For this review, take the finished solid that the model builds, in its own axes (mm). Face numbers are marked on the shaded views. A direction names the side the tool comes from. Give positions to 0.01 mm unless a question says otherwise; leave off trailing zeros. Order: outer loops, then holes, each group sorted by start corner. A loop starts at its lowest first (then second) coordinate and runs counter-clockwise, first axis right, second up. Notation, with made-up numbers: (78, -37.5) -> (96, -37.5) arc R29 ccw to (96, -1.5) -> close; hole circle Ø4 at (36.5, 63.25). An arc over 180 degrees is marked (long way). Return JSON: item names as keys, results as strings. Group by question number.
1) The part is to be moulded in two halves that separate along Y. For the marked faces 6, 7 and 8, say which applies: released by +Y, released by -Y, zero draft, split by the parting line, or undercut.
2) Add section B-B (x = -2.5). Give the boundary of the cut face in (y, z).
3) Add section D-D (y = 15). Give the boundary of the cut face in (x, z), then the cut area to 3 significant figures.
4) For the marked faces 1, 2, 3, 4 and 5, list the 3-axis set-ups (+Z, -Z, +X, -X, +Y, -Y) from which the entire face can be reached by the end or side of a thin tool; tool diameter is ignored.
5) Add section A-A (y = 7). Give the boundary of the cut face in (x, z), then the cut area to 3 significant figures.
6) Add section C-C (z = -5). Give the boundary of the cut face in (x, y), then the cut area to 3 significant figures.
7) To check wall thickness, follow line 1 along X through (y, z) = (-1.25, -5); line 2 along Y through (x, z) = (6, 7); line 3 along Z through (x, y) = (-10, -1.95). State the ranges of each line that lie inside material, in increasing order.
8) Insertion check: P1, Ø9, axis at x = 10, z = -5, coming from the +Y side; P2, Ø11, axis at y = 10, z = 4.5, coming from the +X side; P3, Ø2.5, axis at x = -12, z = -6, coming from the +Y side; P4, Ø4, axis at x = -10, z = -5, coming from the -Y side (1 decimal). Each pin has a flat end and moves straight along its axis. Give the tip position at first contact, or say it passes through.
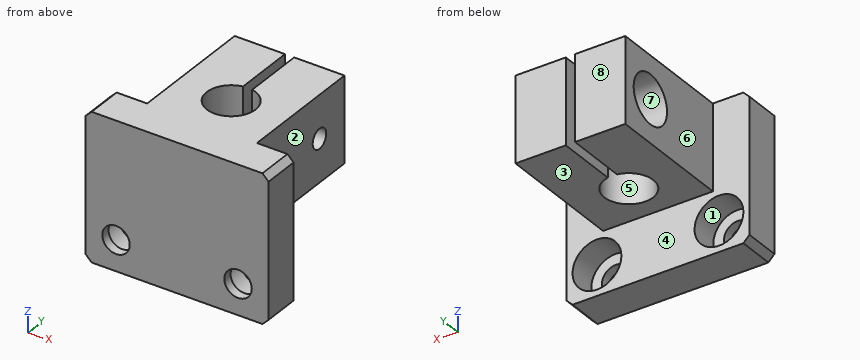
Autodesk Inventor part; units mm, degrees
ref_plane "YZ Plane" through (0, 0, 0) normal (1, 0, 0) x (0, 1, 0)
ref_plane "XZ Plane" through (0, 0, 0) normal (0, 1, 0) x (-1, 0, 0)
ref_plane "XY Plane" through (0, 0, 0) normal (0, 0, 1) x (1, 0, 0)
sketch "スケッチ1" plane through (0, 0, 0) normal (0, 0, 1) x (1, 0, 0)
  line L0 (-9, 21) -> (9, 21)
  line L1 (9, 21) -> (9, 0)
  line L2 (9, 0) -> (-9, 0)
  line L3 (-9, 0) -> (-9, 21)
  point P0 (0, 0)
  point P1 (0, 0)
  dimension "d0" = 18
  dimension "d1" = 21
extrude "押し出し1" add sketch "スケッチ1" along normal blind 14
sketch "スケッチ3" plane through (0, 0, 14) normal (0, 0, 1) x (1, 0, 0)
  line L0 (-9, 21) -> (9, 21)
  point P0 (0, 0)
  point P1 (0, 7)
  point P2 (0, 21)
  dimension "d41" = 14
hole "穴2" at (0, 7, 14) direction (0, 0, -1) diameter 8 end through all
sketch "スケッチ4" plane through (-9, 21, 0) normal (0, 1, 0) x (1, 0, 0)
  line L0 (0, -14) -> (18, -14)
  line L1 (0, 0) -> (18, 0)
  line L2 (8.25, 0) -> (9.75, 0)
  line L3 (9.75, 0) -> (9.75, -14)
  line L4 (9.75, -14) -> (8.25, -14)
  line L5 (8.25, -14) -> (8.25, 0)
  point P0 (9, 0)
  point P1 (9, 0)
  point P2 (9, 0)
  dimension "d21" = 1.5
extrude "押し出し2" cut sketch "スケッチ4" against normal up to surface
sketch "スケッチ5" plane through (-9, 0, 0) normal (-1, 0, 0) x (0, 0, 1)
  line L0 (0, 21) -> (14, 21)
  point P0 (7, 15)
  point P1 (7, 21)
  dimension "d42" = 6
hole "穴3" at (-9, 15, 7) direction (1, 0, 0) diameter 4.5 end up to surface counterbore diameter 8 counterbore depth 4.5
sketch "スケッチ6" plane through (9, 0, 0) normal (1, 0, 0) x (0, 0, -1)
  circle A0 centre (-7, 15) radius 2.25
hole "穴4" at (9, 15, 7) direction (-1, 0, 0) diameter 3.242 end up to surface
sketch "スケッチ9" plane through (-9, 0, 0) normal (0, -1, 0) x (1, 0, 0)
  line L0 (18, 14) -> (0, 14)
  line L1 (18, 0) -> (0, 0)
  line L2 (-6, 14) -> (24, 14)
  line L3 (24, 14) -> (24, -10)
  line L4 (24, -10) -> (-6, -10)
  line L5 (-6, -10) -> (-6, 14)
  point P0 (9, -10)
  point P1 (9, 0)
  dimension "d46" = 30
  dimension "d47" = 24
extrude "押し出し5" add sketch "スケッチ9" along normal blind 6
sketch "スケッチ10" plane through (-9, 0, 0) normal (0, 1, 0) x (1, 0, 0)
  line L0 (24, 10) -> (-6, 10)
  point P0 (9, 0)
  point P1 (-1, 5)
  point P2 (19, 5)
  dimension "d50" = 10
  dimension "d51" = 10
  dimension "d52" = 5
hole "穴5" at (-10, 0, -5) at (10, 0, -5) direction (0, -1, 0) diameter 4.5 end through all counterbore diameter 8 counterbore depth 4.5
chamfer "面取り1" distance 1 angle 45 4 edges at (15, -3, 14) (-15, -3, 14) (-15, -3, -10) (15, -3, -10)
properties part number "06" material "SUS303"
Evaluation:
{
 "1": {"face 6": "zero draft", "face 7": "undercut", "face 8": "released by +Y"},
 "2": {"outline": "(-6, -10) -> (0, -10) -> (0, 0) -> (3.88, 0) -> (3.88, 14) -> (-6, 14) -> close; (10.12, 0) -> (21, 0) -> (21, 14) -> (10.12, 14) -> close; hole circle Ø4.5 at (15, 7)"},
 "3": {"outline": "(-9, 0) -> (-0.75, 0) -> (-0.75, 4.75) -> (-4.5, 4.75) -> (-4.5, 3) -> (-9, 3) -> close; (-9, 11) -> (-4.5, 11) -> (-4.5, 9.25) -> (-0.75, 9.25) -> (-0.75, 14) -> (-9, 14) -> close; (0.75, 0) -> (9, 0) -> (9, 5.38) -> (0.75, 5.38) -> close; (0.75, 8.62) -> (9, 8.62) -> (9, 14) -> (0.75, 14) -> close", "area": "151 mm^2"},
 "4": {"face 1": "+Y", "face 2": "+Z, -Z, +X, +Y", "face 3": "-Z, +X, -X, +Y", "face 4": "-Z, +Y", "face 5": "+Z, -Z"},
 "5": {"outline": "(-9, 0) -> (-4, 0) -> (-4, 14) -> (-9, 14) -> close; (4, 0) -> (9, 0) -> (9, 14) -> (4, 14) -> close", "area": "140 mm^2"},
 "6": {"outline": "(-15, -6) -> (-12.25, -6) -> (-12.25, -4.5) -> (-14, -4.5) -> (-14, 0) -> (-15, 0) -> close; (-7.75, -6) -> (7.75, -6) -> (7.75, -4.5) -> (6, -4.5) -> (6, 0) -> (-6, 0) -> (-6, -4.5) -> (-7.75, -4.5) -> close; (12.25, -6) -> (15, -6) -> (15, 0) -> (14, 0) -> (14, -4.5) -> (12.25, -4.5) -> close", "area": "94.5 mm^2"},
 "7": {"line 1": "-15 to -14, -6 to 6, 14 to 15", "line 2": "-6 to 13.38, 16.62 to 21", "line 3": "-10 to -9, -1 to 14"},
 "8": {"P1": "y = 0", "P2": "x = 9", "P3": "y = -4.5", "P4": "through"}
}
